from build123d import *

# Parameters (mm, degrees)
F0_W     = 115
F0_H     = 50
F1_DEPTH = 80
F2_SIZE  = 50
F3_DEPTH = 15
F4_T     = -1.2
F5_DEPTH = 1.8


with BuildPart() as f1:
    # F0 (on Top) → F1 (new body)
    with BuildSketch(Plane.XY):
        Polygon((58.7, -28), (58.7, -25), (58.7, 26.2), (-58.7, 26.2), (-58.7, -25), (-58.7, -28), (-57.5, -28), (57.5, -28), align=None)
        Rectangle(F0_W, F0_H, mode=Mode.SUBTRACT)
        Rectangle(F0_W, F0_H)
    extrude(amount=F1_DEPTH)

    # F2
    f2_edges = [f1.edges().sort_by_distance(p)[0] for p in [
        (0, 26.2, 80),
    ]]
    chamfer(f2_edges, length=F2_SIZE)

    # F3 (add): a face of the model
    f3_faces = [f1.faces().sort_by_distance(p)[0] for p in [
        (0, -25.9, 80),
    ]]
    extrude(f3_faces, amount=F3_DEPTH)

    # F4
    f4_openings = [f1.faces().sort_by_distance(p)[0] for p in [
        (0, -0.9, 0),
    ]]
    offset(amount=F4_T, openings=f4_openings, kind=Kind.INTERSECTION)

    # F5 (add): a face of the model
    f5_faces = [f1.faces().sort_by_distance(p)[0] for p in [
        (0, -26.8, 46.9),
    ]]
    extrude(f5_faces, amount=F5_DEPTH)


solid = f1.part
Here's how the part is built. I have some questions about the finished solid (model axes, mm). A direction names the side the tool comes from. Round coordinates to 2 decimals unless told otherwise and drop trailing zeros. Order: outer loops, then holes, each group sorted by start corner. A loop starts at its lowest first (then second) coordinate and runs counter-clockwise, first axis right, second up. Notation, with made-up numbers: M 81.5,52 L 94.5,52 A32 cw 94.5,91 Z; hole C -38,17.25 d8. An arc over 180 degrees is marked long. Return JSON: item names as keys, results as strings. Group by question number.
1. If we mould it in two halves opening along X, with no side actions, what happens to faces 3 (the face through (-58.7, -7, 36)), 4 (the face through (1, -23.8, 87)), 5 (the face through (0.805, -0.35, 54.853)), 6 (the face through (-1, -25, 39))? For each: pulls with the +X half, pulls with the -X half, needs draft (parallel to the pull), parting line crosses it, or undercut.
2. I'm going to push flat-ended pins straight in: pin 1 Ø12 at (x, y) = (9.5, 18) entering from -Z; pin 2 Ø4.5 at (x, z) = (-2, 90.5) entering from +Y; pin 3 Ø1 at (x, y) = (11.5, -19.5) entering from -Z. Where does each tip first touch, or does it pass through?
3. On a 3-axis mill with a long thin cutter (end or side, diameter ignored), from which of +Z, -Z, +X, -X, +Y, -Y can I reach the whole of each face in a straight line? I mean faces 1 (the face through (1, 25, 15)), 2 (the face through (1, 26.2, 15)). Say none if no direction works.
4. Please list where these lines run through material, in increasing order: probe 1 along Y at (x, z) = (51, 18); probe 2 along X at (y, z) = (-8, 15.5); probe 3 along Y at (x, z) = (-31, 51).
5. If we section it at A-A on z = 27.5: List the corners of the cut face in (x, y) for me.
6. If we section it at D-D on z = 63.5: List the corners of the cut face in (x, y) for me.
7. If we section it at B-B on x = 25: List the corners of the cut face in (y, z) for me.
8. If we section it at C-C on y = -12: List the corners of the cut face in (x, z) for me, then the cut area to 3 significant figures.
Reply:
{
 "1": {"face 3": "pulls with the -X half", "face 4": "needs draft", "face 5": "undercut", "face 6": "undercut"},
 "2": {"pin 1": "z = 30.5", "pin 2": "y = -23.8", "pin 3": "z = 73.5"},
 "3": {"face 1": "-Z", "face 2": "+Z, -Z, +X, -X, +Y"},
 "4": {"probe 1": "-28 to -25, 25 to 26.2", "probe 2": "-58.7 to -57.5, 57.5 to 58.7", "probe 3": "-28 to -25, 3.5 to 5.2"},
 "5": {"outline": "M -58.7,-28 L 58.7,-28 L 58.7,26.2 L -58.7,26.2 Z; hole M -57.5,-25 L 57.5,-25 L 57.5,25 L -57.5,25 Z"},
 "6": {"outline": "M -58.7,-28 L 58.7,-28 L 58.7,-7.3 L -58.7,-7.3 Z; hole M -57.5,-25 L 57.5,-25 L 57.5,-9 L -57.5,-9 Z"},
 "7": {"outline": "M -28,0 L -25,0 L -25,79.5 L 25,29.5 L 25,0 L 26.2,0 L 26.2,30 L -23.8,80 L -23.8,95 L -28,95 Z"},
 "8": {"outline": "M -58.7,0 L -57.5,0 L -57.5,66.5 L 57.5,66.5 L 57.5,0 L 58.7,0 L 58.7,68.2 L -58.7,68.2 Z", "area": "359 mm^2"}
}
